Design review of the part built by this model. Coordinates are the model's own, in mm. A direction names the side the tool comes from. Coordinates: 2 decimals unless noted, no trailing zeros. Write each loop counter-clockwise with the first axis right and the second up, starting at its lowest first coordinate (ties: lowest second). Pieces come first, ordered by that corner, then holes. Notation, with made-up numbers: (52.25, 44) - (62.25, 44) arc R15 cw to (62.25, 57) - close; hole circle Ø7 at (41.25, 15). An arc over 180 degrees is marked (long way). Use a Markdown table: item, result.
from build123d import *

# Parameters (mm, degrees)
F1_DEPTH = 3
F2_DEPTH = 57
F6_DEPTH = 26
F7_R     = 3.379899
F8_R     = 2.897056


with BuildPart() as f1:
    # F0 (on Top) → F1 (new body)
    with BuildSketch(Plane.XY):
        with BuildLine():
            Line((-55.075931, -7.509255), (-55.075931, 42.226299))
            Line((-55.075931, 42.226299), (-36.499178, 42.226299))
            ThreePointArc((-36.499178, 42.226299), (-154.89147, 58.109982), (-55.075931, -7.509255))
        make_face()
        with BuildLine():
            Line((-36.499178, 42.226299), (-55.075931, 42.226299))
            Line((-55.075931, 42.226299), (-55.075931, -7.509255))
            ThreePointArc((-55.075931, -7.509255), (-41.150625, 12.660964), (-36.247192, 36.675714))
            ThreePointArc((-36.247192, 36.675714), (-36.310221, 39.453865), (-36.499178, 42.226299))
        make_face()
        with BuildLine():
            Line((-5.075931, 42.226299), (-36.499178, 42.226299))
            ThreePointArc((-36.499178, 42.226299), (-36.310221, 39.453865), (-36.247192, 36.675714))
            ThreePointArc((-36.247192, 36.675714), (-41.150625, 12.660964), (-55.075931, -7.509255))
            Line((-55.075931, -7.509255), (-55.075931, -17.773701))
            Line((-55.075931, -17.773701), (-5.075931, -17.773701))
            Line((-5.075931, -17.773701), (-5.075931, 42.226299))
        make_face()
    extrude(amount=F1_DEPTH)

    # F0 (on Top) → F2 (cut)
    with BuildSketch(Plane.XY):
        with BuildLine():
            Line((-36.499178, 42.226299), (-55.075931, 42.226299))
            Line((-55.075931, 42.226299), (-55.075931, -7.509255))
            ThreePointArc((-55.075931, -7.509255), (-41.150625, 12.660964), (-36.247192, 36.675714))
            ThreePointArc((-36.247192, 36.675714), (-36.310221, 39.453865), (-36.499178, 42.226299))
        make_face()
        with BuildLine():
            Line((-55.075931, -7.509255), (-55.075931, 42.226299))
            Line((-55.075931, 42.226299), (-36.499178, 42.226299))
            ThreePointArc((-36.499178, 42.226299), (-154.89147, 58.109982), (-55.075931, -7.509255))
        make_face()
    extrude(amount=F2_DEPTH, mode=Mode.SUBTRACT)

    # F3: F1 across face


with BuildPart() as f1_1:
    add(f1.part)
    add(f1.part.mirror(Plane(origin=(-5.075931, 12.226299, 1.5), x_dir=(0, 1, 0), z_dir=(1, 0, 0))))

    # F4: F1 across face


with BuildPart() as f1_2:
    add(f1_1.part)
    add(f1_1.part.mirror(Plane(origin=(-5.075931, -17.773701, 1.5), x_dir=(1, 0, 0), z_dir=(0, -1, 0))))

    # F5 (on face) → F6 (join)
    with BuildSketch(Plane.XY.offset(3)):
        Polygon((-11.076178, -70.267022), (-5.076178, -70.267022), (0.923822, -70.267022), (0.923822, -64.267022), (-5.076178, -64.267022), (-11.076178, -64.267022), align=None)
    extrude(amount=F6_DEPTH)

    # F7
    f7_edges = [f1_2.edges().sort_by_distance(p)[0] for p in [
        (-5.076178, -70.267022, 29),
    ]]
    fillet(f7_edges, radius=F7_R)

    # F8
    f8_edges = [f1_2.edges().sort_by_distance(p)[0] for p in [
        (-5.076178, -64.267022, 29),
    ]]
    fillet(f8_edges, radius=F8_R)


solid = f1_2.part
(1) For L1, parallel to Z at x = 14.5, y = -7; L2, parallel to X at y = -69.5, z = 11.5; L3, parallel to Y at x = -7, z = 5.25, list the stretches that pass through material, from the lowest coordinate up. Write a range as from..to.
Determined:
| item | result |
|---|---|
| L1 | 0..3 |
| L2 | -11.08..0.92 |
| L3 | -70.27..-64.27 |
(2) For pin 1 (3 mm diameter, centred on x = -14.5, z = 17.5, fed in from +Y); pin 2 (8 mm diameter, centred on y = 5, z = 4.5, fed in from +X); pin 3 (6.5 mm diameter, centred on y = -68, z = 15.5, fed in from +X); pin 4 (6 mm diameter, centred on x = 29.5, y = -56.5, fed in from +Z), all flat-tipped, find the tip position at first contact; note any pin that passes through.
Determined:
| item | result |
|---|---|
| pin 1 | through |
| pin 2 | x = 37.35 |
| pin 3 | x = 0.92 |
| pin 4 | z = 3 |
(3) Take a section at A-A on z = 12.75. Write out the cut boundary in (x, y), and give its area (3 significant figures).
Determined:
| item | result |
|---|---|
| outline | (-11.08, -70.27) - (0.92, -70.27) - (0.92, -64.27) - (-11.08, -64.27) - close |
| area | 72.0 mm2 |
(4) Machinability: for faces 4 (the flat face through (-5, -64.267, 14)), 5 (the flat face through (0.924, -67, 16)), 6 (the cylindrical face through (-36.31, -74.96, 1.48)), 7 (the cylindrical face through (26.157, 39.415, 1.479)), which of the approach directions +Z, -Z, +X, -X, +Y, -Y give a long, thin tool a straight path to every point of the face, cutting with its end or side? Answer none if there is none.
Determined:
| item | result |
|---|---|
| face 4 | +Z, +X, -X, +Y |
| face 5 | +Z, +X, +Y, -Y |
| face 6 | +Z, -Z, -X |
| face 7 | +Z, -Z, +X |
(5) Take a section at B-B on x = 36.5. Write out the cut boundary in (y, z), and give its area (3 significant figures).
Determined:
| item | result |
|---|---|
| outline | (-38.07, 0) - (2.52, 0) - (2.52, 3) - (-38.07, 3) - close |
| area | 122 mm2 |
(6) Draft analysis for pull direction Y (two halves, no side actions). For faces 1 (the cylindrical face through (26.157, -74.962, 1.479)), 2 (the flat face through (-5, -70.267, 14)), 3 (the flat face through (-11.076, -67, 16)), state which applies: +Y half, -Y half, draft (parallel to the pull), parting line (faces both ways), or undercut.
Determined:
| item | result |
|---|---|
| face 1 | undercut |
| face 2 | -Y half |
| face 3 | draft |
